```python
from build123d import *

# Parameters (mm, degrees)
SKETCH1_R               = 3
BOSS_EXTRUDE1_DEPTH     = 95
SKETCH2_R               = 1.7
CUT_EXTRUDE1_DEPTH      = 96.094689652
CHAMFER1_SIZE           = 0.3
CUT_EXTRUDE2_DEPTH      = 96.094689652
CUT_EXTRUDE2_DEPTH_BACK = 96.094689652
SKETCH3_R               = 1.25


with BuildPart() as part:
    # Sketch1 → Boss-Extrude1 (new body)
    with BuildSketch(Plane(origin=(0, 0, 0), x_dir=(1, 0, 0), z_dir=(0, 1, 0))):
        with Locations(Location((0, 0, 0), (0, 0, 270))):
            Circle(SKETCH1_R)
    extrude(amount=BOSS_EXTRUDE1_DEPTH)

    # Sketch2 → Cut-Extrude1 (cut, through all)
    with BuildSketch(Plane(origin=(0, 95, 0), x_dir=(1, 0, 0), z_dir=(0, 1, 0))):
        with Locations(Location((0, 0, 0), (0, 0, 270))):
            Circle(SKETCH2_R)
    extrude(amount=-CUT_EXTRUDE1_DEPTH, mode=Mode.SUBTRACT)

    # Chamfer1
    chamfer1_edges = [part.edges().sort_by_distance(p)[0] for p in [
        (0, 0, -3),
    ]]
    chamfer(chamfer1_edges, length=CHAMFER1_SIZE)

    # Sketch3 → Cut-Extrude2 (cut, two sides: drawn at the far end of the back side and taken through both)
    with BuildSketch(Plane(origin=(0, 0, 0), x_dir=(0, 0, -1), z_dir=(1, 0, 0)).offset(-CUT_EXTRUDE2_DEPTH_BACK)):
        Circle(SKETCH3_R)
    extrude(amount=CUT_EXTRUDE2_DEPTH + CUT_EXTRUDE2_DEPTH_BACK, mode=Mode.SUBTRACT)


solid = part.part
```
Check sheet for the modelled part. Datum: model origin and axes. Units: mm. Round coordinates to 2 decimals unless told otherwise and drop trailing zeros. Loops run counter-clockwise (first coordinate to the right, second up) from the corner with the lowest first, then second, coordinate; pieces in that order, holes last. Notation, with made-up numbers: (71, 36.5) - (88, 36.5) arc R24 cw to (88, 46.5) - close; hole circle Ø10 at (36.25, 8). An arc over 180 degrees is marked (long way). Write item = value, one per line. Start each with the question number.
Q1. Release check for a two-part mould opening along X. For faces 1 (the face through (0, 0, 2)), 2 (the face through (0.9, 46.99, 2.86)), 3 (the face through (-1.66, 48.16, -0.37)) record: pulls with the +X half, pulls with the -X half, needs draft (parallel to the pull), parting line crosses it, or undercut.
Q2. Depth check by flat-ended pin: P1, Ø1, axis at y = 23.5, z = -2, coming from the +X side. Enter the tip coordinate at first touch or a pass-through.
Q3. Section check B-B (z = 0). Record the boundary of the cut face in (x, y).
Q4. Thickness scan on L1, parallel to X at y = 19.5, z = 0; L2, parallel to Z at x = -1.25, y = 85; L3, parallel to Z at x = -1.5, y = 82. Record the ranges inside material, lowest first.
Q5. Section check A-A (x = 0). Record the boundary of the cut face in (y, z).
Q6. Section check C-C (y = 49). Record the boundary of the cut face in (x, z).
Derived:
q1.face_1 = needs draft
q1.face_2 = parting line crosses it
q1.face_3 = undercut
q2.P1 = 2.6
q3.outline = (-3, 1.25) - (-1.7, 1.25) - (-1.7, 95) - (-3, 95) - close; (1.7, 1.25) - (3, 1.25) - (3, 95) - (1.7, 95) - close
q4.L1 = -3 to -1.7, 1.7 to 3
q4.L2 = -2.73 to -1.15, 1.15 to 2.73
q4.L3 = -2.6 to -0.8, 0.8 to 2.6
q5.outline = (0, -2.7) - (0.3, -3) - (95, -3) - (95, -1.7) - (0, -1.7) - close; (0, 1.7) - (95, 1.7) - (95, 3) - (0.3, 3) - (0, 2.7) - close
q6.outline = circle Ø6 at (0, 0); hole circle Ø3.4 at (0, 0)
